The listing builds one solid part. Answer for the finished solid, in the listing's coordinates (mm). Face numbers are marked on the shaded views. A direction names the side the tool comes from. Give positions to 0.01 mm unless a question says otherwise; leave off trailing zeros. Order: outer loops, then holes, each group sorted by start corner. A loop starts at its lowest first (then second) coordinate and runs counter-clockwise, first axis right, second up.
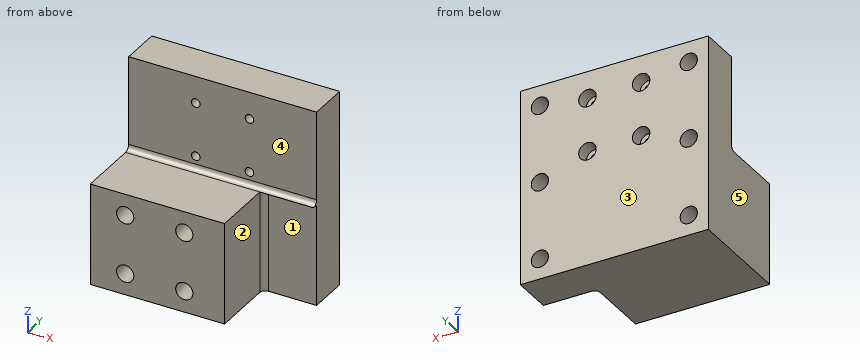
```python
from build123d import *

# Parameters (mm, degrees)
SKETCH1_W           = 70
SKETCH1_H           = 40
SKETCH1_R           = 1.6
BOSS_EXTRUDE1_DEPTH = 15
SKETCH2_R           = 3.25
CUT_EXTRUDE1_DEPTH  = 5
SKETCH3_W           = 70
SKETCH3_H           = 37.813008
BOSS_EXTRUDE2_DEPTH = 39.896897
FILLET1_R           = 2
SKETCH4_R           = 3.2
CUT_EXTRUDE2_DEPTH  = 8
SKETCH5_R           = 3.2
CUT_EXTRUDE3_DEPTH  = 10
CUT_EXTRUDE4_REACH  = 76.873
SKETCH7_W           = 20
SKETCH7_H           = 37.813008
FILLET2_R           = 2


with BuildPart() as part:
    # Sketch1 → Boss-Extrude1 (new body)
    with BuildSketch(Plane(origin=(0, 0, 0), x_dir=(1, 0, 0), z_dir=(0, 1, 0))):
        Rectangle(SKETCH1_W, SKETCH1_H)
        with Locations(Location((10, 10, 0), (0, 0, 270))):
            Circle(SKETCH1_R, mode=Mode.SUBTRACT)
        with Locations(Location((10, -10, 0), (0, 0, 270))):
            Circle(SKETCH1_R, mode=Mode.SUBTRACT)
        with Locations(Location((-10, -10, 0), (0, 0, 270))):
            Circle(SKETCH1_R, mode=Mode.SUBTRACT)
        with Locations(Location((-10, 10, 0), (0, 0, 270))):
            Circle(SKETCH1_R, mode=Mode.SUBTRACT)
    extrude(amount=BOSS_EXTRUDE1_DEPTH)

    # Sketch2 → Cut-Extrude1 (cut)
    with BuildSketch(Plane(origin=(0, 15, 0), x_dir=(1, 0, 0), z_dir=(0, 1, 0))):
        with Locations(Location((10, 10, 0), (0, 0, 270))):
            Circle(SKETCH2_R)
        with Locations(Location((10, -10, 0), (0, 0, 270))):
            Circle(SKETCH2_R)
        with Locations(Location((-10, -10, 0), (0, 0, 270))):
            Circle(SKETCH2_R)
        with Locations(Location((-10, 10, 0), (0, 0, 270))):
            Circle(SKETCH2_R)
    extrude(amount=-CUT_EXTRUDE1_DEPTH, mode=Mode.SUBTRACT)

    # Sketch3 → Boss-Extrude2 (add)
    with BuildSketch(Plane(origin=(0, 15, 0), x_dir=(1, 0, 0), z_dir=(0, 1, 0))):
        with Locations((0, 33.906504)):
            Rectangle(SKETCH3_W, SKETCH3_H)
    extrude(amount=-BOSS_EXTRUDE2_DEPTH)

    # Fillet1
    fillet1_edges = [part.edges().sort_by_distance(p)[0] for p in [
        (0, 0, -15),
    ]]
    fillet(fillet1_edges, radius=FILLET1_R)

    # Sketch4 → Cut-Extrude2 (cut)
    with BuildSketch(Plane(origin=(0, 15, 0), x_dir=(1, 0, 0), z_dir=(0, 1, 0))):
        with Locations(Location((27.721774771, 45.242301259, 0), (0, 0, 270))):
            Circle(SKETCH4_R)
        with Locations(Location((-27.721774771, 45.242301259, 0), (0, 0, 90))):
            Circle(SKETCH4_R)
        with Locations(Location((-27.721774771, -12.429293259, 0), (0, 0, 270))):
            Circle(SKETCH4_R)
        with Locations(Location((27.721774771, -12.429293259, 0), (0, 0, 90))):
            Circle(SKETCH4_R)
        with Locations(Location((27.721774771, 16.406504, 0), (0, 0, 270))):
            Circle(SKETCH4_R)
        with Locations(Location((-27.721774771, 16.406504, 0), (0, 0, 90))):
            Circle(SKETCH4_R)
    extrude(amount=-CUT_EXTRUDE2_DEPTH, mode=Mode.SUBTRACT)

    # Sketch5 → Cut-Extrude3 (cut)
    with BuildSketch(Plane.XZ.offset(24.896897)):
        with Locations(Location((0, -22.906504, 0), (0, 0, 270))):
            Circle(SKETCH5_R)
        with Locations(Location((0, -44.906504, 0), (0, 0, 90))):
            Circle(SKETCH5_R)
        with Locations(Location((-22, -22.906504, 0), (0, 0, 270))):
            Circle(SKETCH5_R)
        with Locations(Location((-22, -44.906504, 0), (0, 0, 90))):
            Circle(SKETCH5_R)
    extrude(amount=-CUT_EXTRUDE3_DEPTH, mode=Mode.SUBTRACT)

    # Cut-Extrude4: up to this face of the body (flat: up to its plane)
    cut_extrude4_end = Plane(part.part.faces().sort_by_distance((0, 0, 3.549430676))[0])
    # Sketch7 → Cut-Extrude4 (cut, up to the picked face)
    with BuildSketch(Plane.XZ.offset(24.896897), mode=Mode.PRIVATE) as cut_extrude4_sk1:
        with Locations((25, -33.906504)):
            Rectangle(SKETCH7_W, SKETCH7_H)
    cut_extrude4_tool1 = split(extrude(cut_extrude4_sk1.sketch, amount=-CUT_EXTRUDE4_REACH, mode=Mode.PRIVATE), bisect_by=cut_extrude4_end, keep=Keep.BOTH, mode=Mode.PRIVATE)
    add(cut_extrude4_tool1.solids().sort_by(Axis((25, -24.896897, -33.906504), (0, 1, 0)))[0], mode=Mode.SUBTRACT)

    # Fillet2
    fillet2_edges = [part.edges().sort_by_distance(p)[0] for p in [
        (15, 0, -33.906504),
    ]]
    fillet(fillet2_edges, radius=FILLET2_R)


solid = part.part
```
1) Find section B-B (z = -30). Write down the section's boundary in (x, y), then the cut area to 3 significant figures.
Geometry says:
outline: (-35, -24.9) - (15, -24.9) - (15, -2) arc R2 cw to (17, 0) - (35, 0) - (35, 15) - (-35, 15) - close
area: 2,300 mm2
2) Find section C-C (x = 0). Write down the section's boundary in (y, z), then the cut area to 3 significant figures.
Geometry says:
outline: (-24.9, -52.81) - (15, -52.81) - (15, 20) - (0, 20) - (0, -13) arc R2 cw to (-2, -15) - (-24.9, -15) - (-24.9, -19.71) - (-14.9, -19.71) - (-14.9, -26.11) - (-24.9, -26.11) - (-24.9, -41.71) - (-14.9, -41.71) - (-14.9, -48.11) - (-24.9, -48.11) - close
area: 1,910 mm2
3) Straight lines are drawn through the part: probe 1 along X at (y, z) = (12.25, -10); probe 2 along Z at (x, y) = (10, 3); probe 3 along Z at (x, y) = (-1, -16.5). For each, find the intervals that lie inside material, in ascending order.
Geometry says:
probe 1: x = -35 to -13.25, -6.75 to 6.75, 13.25 to 35
probe 2: z = -52.81 to -11.6, -8.4 to 8.4, 11.6 to 20
probe 3: z = -52.81 to -47.95, -41.87 to -25.95, -19.87 to -15
4) Find section A-A (x = 10). Write down the section's boundary in (y, z), then the cut area to 3 significant figures.
Geometry says:
outline: (-24.9, -52.81) - (15, -52.81) - (15, -13.25) - (10, -13.25) - (10, -11.6) - (0, -11.6) - (0, -13) arc R2 cw to (-2, -15) - (-24.9, -15) - close; (0, -8.4) - (10, -8.4) - (10, -6.75) - (15, -6.75) - (15, 6.75) - (10, 6.75) - (10, 8.4) - (0, 8.4) - close; (0, 11.6) - (10, 11.6) - (10, 13.25) - (15, 13.25) - (15, 20) - (0, 20) - close
area: 1,910 mm2
5) Given P1, Ø3, axis at x = -27.5, z = 13.5, coming from the +Y side; P2, Ø1.5, axis at y = -10.5, z = -21, coming from the +X side; P3, Ø3.5, axis at x = -10, z = -10, coming from the -Y side; P4, Ø10, axis at x = -27.72, z = -16.41, coming from the +Y side, each flat-ended and moving along its own axis, determine where each tip first touches the part or whether it passes through.
Geometry says:
P1: stops at y = 7
P2: stops at x = 15
P3: stops at y = 0
P4: stops at y = 15
6) A tool of negligible diameter and unlimited length cuts with its end or side. For the marked faces 1, 2, 3, 4 and 5, from which of +Z, -Z, +X, -X, +Y, -Y can it reach the whole face along a straight path? Write none if from no direction.
Geometry says:
face 1: -Z, +X, -Y
face 2: +Z, -Z, +X, -Y
face 3: +Z, -Z, +X, -X, +Y
face 4: +Z, +X, -X, -Y
face 5: +Z, -Z, -X, +Y, -Y
7) Find section D-D (y = -7). Write down the section's boundary in (x, z).
Geometry says:
outline: (-35, -52.81) - (15, -52.81) - (15, -15) - (-35, -15) - close
